Work out the finished part from the listing and answer in its coordinate system (mm). A direction names the side the tool comes from. Coordinates: 2 decimals unless noted, no trailing zeros. Loops run counter-clockwise (first coordinate to the right, second up) from the corner with the lowest first, then second, coordinate; pieces in that order, holes last.
```python
from build123d import *

# Parameters (mm, degrees)
F0_W           = 35
F0_H           = 17
F1_DEPTH       = 47
F2_W           = 30
F2_H           = 13
F2_W_2         = 1
F3_DEPTH       = 45
F2_W_3         = 2
F2_H_2         = 1
F4_DEPTH       = 46
F6_D           = 3
F6_DEPTH       = 3
F6_CSINK_D     = 6
F6_CSINK_ANGLE = 90
F6_TIP         = 0.9012909285
F8_D           = 3
F8_DEPTH       = 3
F8_CSINK_D     = 6
F8_CSINK_ANGLE = 90
F8_TIP         = 0.9012909285


with BuildPart() as f1:
    # F0 (on Right) → F1 (new body)
    with BuildSketch(Plane.YZ):
        Rectangle(F0_W, F0_H)
    extrude(amount=F1_DEPTH)

    # F2 (on face) → F3 (cut)
    with BuildSketch(Plane.YZ.offset(47)):
        with Locations((0.5, 0)):
            Rectangle(F2_W, F2_H)
        with Locations((-17, 0)):
            Rectangle(F2_W_2, F2_H)
    extrude(amount=-F3_DEPTH, mode=Mode.SUBTRACT)

    # F2 (on face) → F4 (cut)
    with BuildSketch(Plane.YZ.offset(47)):
        with Locations((-15.5, 0)):
            Rectangle(F2_W_3, F2_H)
        with Locations((-15.5, 7)):
            Rectangle(F2_W_3, F2_H_2)
        with Locations((-15.5, -7)):
            Rectangle(F2_W_3, F2_H_2)
    extrude(amount=-F4_DEPTH, mode=Mode.SUBTRACT)

    # F6
    with Locations(Plane.XY.offset(8.5)):
        with Locations((43.5, 0)):
            CounterSinkHole(F6_D / 2, F6_CSINK_D / 2, depth=F6_DEPTH, counter_sink_angle=F6_CSINK_ANGLE)
            with Locations((0, 0, -(F6_DEPTH + F6_TIP / 2))):  # 118° drill point
                Cone(0, F6_D / 2, F6_TIP, mode=Mode.SUBTRACT)

    # F8
    with Locations(Plane(origin=(0, 0, -8.5), x_dir=(1, 0, 0), z_dir=(0, 0, -1))):
        with Locations((43.5, 0)):
            CounterSinkHole(F8_D / 2, F8_CSINK_D / 2, depth=F8_DEPTH, counter_sink_angle=F8_CSINK_ANGLE)
            with Locations((0, 0, -(F8_DEPTH + F8_TIP / 2))):  # 118° drill point
                Cone(0, F8_D / 2, F8_TIP, mode=Mode.SUBTRACT)


solid = f1.part
```
1. Each of these flat-tipped pins is pushed along its axis until it touches: P1, Ø3.5, axis at x = 43.5, y = 0, coming from the +Z side; P2, Ø0.6, axis at y = -15, z = -0.5, coming from the +X side; P3, Ø4, axis at x = 29.5, z = 1.5, coming from the -Y side. Where does it stop, or does it pass through?
2. A cutting plane is placed at A-A, the plane x = 43.5. Give the vertices of the cut face in (y, z), then the cut area to 4 significant figures.
3. Determine the mould class of faces 1 (the flat face through (25, -17, -6.5)), 2 (the flat face through (25, 15.5, 0)), 3 (the flat face through (1, -16, 0)), 4 (the cylindrical face through (45, -0.07, -6.75)) for opening direction Y: released by +Y, released by -Y, zero draft, split by the parting line, or undercut.
4. A cutting plane is placed at D-D, the plane x = 10.5. Give the vertices of the cut face in (y, z), then the cut area to 3 significant figures.
5. Straight lines are drawn through the part: probe 1 along Y at (x, z) = (43.5, -6.8); probe 2 along Z at (x, y) = (21, 13); probe 3 along Z at (x, y) = (27, -16). For each, find the intervals that lie inside material, in ascending order.
6. For faces 5 (the flat face through (24, -16, 7.5)), 6 (the flat face through (25, -17, 6.5)), 7 (the flat face through (23, 17.5, 0)), determine the directions among +Z, -Z, +X, -X, +Y, -Y from which every point of the face is accessible in a straight line to the end or side of a thin tool.
7. A cutting plane is placed at B-B, the plane y = 0. Give the vertices of the cut face in (x, z).
8. A cutting plane is placed at C-C, the plane z = -3.5. Give the vertices of the cut face in (x, y).
Answers below:
1. P1: stops at z = 7.25
1. P2: stops at x = 1
1. P3: stops at y = 15.5
2. outline: (-17.5, -8.5) - (-3, -8.5) - (-1.5, -7) - (-1.5, -6.5) - (-14.5, -6.5) - (-14.5, -7.5) - (-16.5, -7.5) - (-16.5, -6.5) - (-17.5, -6.5) - close; (-17.5, 6.5) - (-16.5, 6.5) - (-16.5, 7.5) - (-14.5, 7.5) - (-14.5, 6.5) - (-1.5, 6.5) - (-1.5, 7) - (-3, 8.5) - (-17.5, 8.5) - close; (1.5, -7) - (3, -8.5) - (17.5, -8.5) - (17.5, 8.5) - (3, 8.5) - (1.5, 7) - (1.5, 6.5) - (15.5, 6.5) - (15.5, -6.5) - (1.5, -6.5) - close
2. area: 145.5 mm2
3. face 1: zero draft
3. face 2: released by -Y
3. face 3: undercut
3. face 4: undercut
4. outline: (-17.5, -8.5) - (17.5, -8.5) - (17.5, 8.5) - (-17.5, 8.5) - (-17.5, 6.5) - (-16.5, 6.5) - (-16.5, 7.5) - (-14.5, 7.5) - (-14.5, 6.5) - (15.5, 6.5) - (15.5, -6.5) - (-14.5, -6.5) - (-14.5, -7.5) - (-16.5, -7.5) - (-16.5, -6.5) - (-17.5, -6.5) - close
4. area: 162 mm2
5. probe 1: y = -17.5 to -16.5, -14.5 to -1.5, 1.5 to 17.5
5. probe 2: z = -8.5 to -6.5, 6.5 to 8.5
5. probe 3: z = -8.5 to -7.5, 7.5 to 8.5
6. face 5: +X
6. face 6: +X, -Y
6. face 7: +Z, -Z, +X, -X, +Y
7. outline: (0, -8.5) - (40.5, -8.5) - (42, -7) - (42, -6.5) - (2, -6.5) - (2, 6.5) - (42, 6.5) - (42, 7) - (40.5, 8.5) - (0, 8.5) - close; (45, -7) - (46.5, -8.5) - (47, -8.5) - (47, -6.5) - (45, -6.5) - close; (45, 6.5) - (47, 6.5) - (47, 8.5) - (46.5, 8.5) - (45, 7) - close
8. outline: (0, -17.5) - (2, -17.5) - (2, -16.5) - (1, -16.5) - (1, -14.5) - (2, -14.5) - (2, 15.5) - (47, 15.5) - (47, 17.5) - (0, 17.5) - close
